```python
from build123d import *

# Parameters (mm, degrees)
SKETCH1_W           = 164.056213182
SKETCH1_H           = 67.71790731
BOSS_EXTRUDE1_DEPTH = 10
SKETCH2_R           = 5.733448678
CUT_EXTRUDE1_DEPTH  = 10
SKETCH4_R           = 6.106577878
CUT_EXTRUDE2_DEPTH  = 10
SKETCH6_R           = 16.472289059
CUT_EXTRUDE3_DEPTH  = 10


with BuildPart() as part:
    # Sketch1 → Boss-Extrude1 (new body)
    with BuildSketch(Plane(origin=(0, 0, 0), x_dir=(1, 0, 0), z_dir=(0, 1, 0))):
        Rectangle(SKETCH1_W, SKETCH1_H)
    extrude(amount=BOSS_EXTRUDE1_DEPTH)

    # Sketch2 → Cut-Extrude1 (cut)
    with BuildSketch(Plane(origin=(0, 10, 0), x_dir=(1, 0, 0), z_dir=(0, 1, 0))):
        with Locations(Location((-40.043133624, 0, 0), (0, 0, 270))):
            Circle(SKETCH2_R)
    extrude(amount=-CUT_EXTRUDE1_DEPTH, mode=Mode.SUBTRACT)

    # Sketch4 → Cut-Extrude2 (cut)
    with BuildSketch(Plane(origin=(0, 10, 0), x_dir=(1, 0, 0), z_dir=(0, 1, 0))):
        with Locations(Location((44.848309659, 0, 0), (0, 0, 270))):
            Circle(SKETCH4_R)
    extrude(amount=-CUT_EXTRUDE2_DEPTH, mode=Mode.SUBTRACT)

    # Sketch6 → Cut-Extrude3 (cut)
    with BuildSketch(Plane(origin=(0, 10, 0), x_dir=(1, 0, 0), z_dir=(0, 1, 0))):
        with Locations(Location((0, 0, 0), (0, 0, 270))):
            Circle(SKETCH6_R)
    extrude(amount=-CUT_EXTRUDE3_DEPTH, mode=Mode.SUBTRACT)


solid = part.part
```
Design review of the part built by this model. Coordinates are the model's own, in mm. Give positions to 0.01 mm unless a question says otherwise; leave off trailing zeros. Order: outer loops, then holes, each group sorted by start corner. A loop starts at its lowest first (then second) coordinate and runs counter-clockwise, first axis right, second up. Notation, with made-up numbers: M 83.25,-7 L 94.25,-7 A10 ccw 94.25,4 Z; hole C 25.5,-36.75 d4. An arc over 180 degrees is marked long. One line per question, with ' | ' between items. Start each with the question number.
Q1. The part is to be moulded in two halves that separate along X. For faces 1 (the face through (82.028, 5, 0)), 2 (the face through (50.903, 5.07, -0.795)), 3 (the face through (17, 0, 0)), 4 (the face through (13.889, 5.07, 8.855)), say which applies: +X half, -X half, draft (parallel to the pull), parting line (faces both ways), or undercut.
Q2. We need section A-A (x = 0). Write out the cut boundary in (y, z).
Q3. We need section B-B (z = 0). Write out the cut boundary in (x, y), plus the area to 3 significant figures.
Q4. For L1, parallel to X at y = 2.75, z = 0; L2, parallel to X at y = 8, z = -11; L3, parallel to X at y = 8.25, z = -15, list the stretches that pass through material, from the lowest coordinate up. Write a range as [from, to].
Q5. We need section C-C (y = 5.5). Write out the cut boundary in (x, z), plus the area to 3 significant figures.
Q6. We need section D-D (z = -10). Write out the cut boundary in (x, y).
Returned:
1) face 1: +X half | face 2: undercut | face 3: draft | face 4: undercut
2) outline: M 0,-33.86 L 10,-33.86 L 10,-16.47 L 0,-16.47 Z; M 0,16.47 L 10,16.47 L 10,33.86 L 0,33.86 Z
3) outline: M -82.03,0 L -45.78,0 L -45.78,10 L -82.03,10 Z; M -34.31,0 L -16.47,0 L -16.47,10 L -34.31,10 Z; M 16.47,0 L 38.74,0 L 38.74,10 L 16.47,10 Z; M 50.95,0 L 82.03,0 L 82.03,10 L 50.95,10 Z | area: 1,070 mm2
4) L1: [-82.03, -45.78], [-34.31, -16.47], [16.47, 38.74], [50.95, 82.03] | L2: [-82.03, -12.26], [12.26, 82.03] | L3: [-82.03, -6.81], [6.81, 82.03]
5) outline: M -82.03,-33.86 L 82.03,-33.86 L 82.03,33.86 L -82.03,33.86 Z; hole C -40.04,0 d11.47; hole C 0,0 d32.94; hole C 44.85,0 d12.21 | area: 10,000 mm2
6) outline: M -82.03,0 L -13.09,0 L -13.09,10 L -82.03,10 Z; M 13.09,0 L 82.03,0 L 82.03,10 L 13.09,10 Z
